For this review, take the finished solid that the model builds, in its own axes (mm). Face numbers are marked on the shaded views. A direction names the side the tool comes from. Round coordinates to 2 decimals unless told otherwise and drop trailing zeros. Loops run counter-clockwise (first coordinate to the right, second up) from the corner with the lowest first, then second, coordinate; pieces in that order, holes last. Notation, with made-up numbers: M 51.25,5.25 L 70.25,5.25 A22 cw 70.25,26.25 Z; hole C -25,43.25 d11. An arc over 180 degrees is marked long. Write item = value, one per line. Start each with the question number.
```python
from build123d import *

# Parameters (mm, degrees)
F0_R     = 3.78
F1_DEPTH = 6.88
F2_R     = 3.1
F3_DEPTH = 4.45
F4_R     = 2.5
F5_DEPTH = 11.6


# Not quite as in the source:
# - a fillet or chamfer that OpenCascade refuses, or shapes differently, is made with other operations: its cross-section is extruded or revolved along the edge and cut away or added


with BuildPart() as f1:
    # F0 (on Top) → F1 (new body)
    with BuildSketch(Plane.XY):
        Circle(F0_R)
    extrude(amount=F1_DEPTH)

    # F2 (on face) → F3 (join)
    with BuildSketch(Plane(origin=(0, 0, 0), x_dir=(1, 0, 0), z_dir=(0, 0, -1))):
        Circle(F2_R)
    extrude(amount=F3_DEPTH)

    # F4 (on face) → F5 (cut)
    with BuildSketch(Plane.XY.offset(6.88)):
        Circle(F4_R)
    extrude(amount=-F5_DEPTH, mode=Mode.SUBTRACT)

    # F6: chamfer of 1.4 on 1 edges, made by hand

    # F6_s1 → F6_t2 (revolve, cut)
    with BuildSketch(Plane.XZ):
        Polygon((3.78, 5.48), (2.38, 6.88), (3.78, 6.88), align=None)
    revolve(axis=Axis((0, 0, 6.88), (0, 0, 1)), mode=Mode.SUBTRACT)


solid = f1.part
```
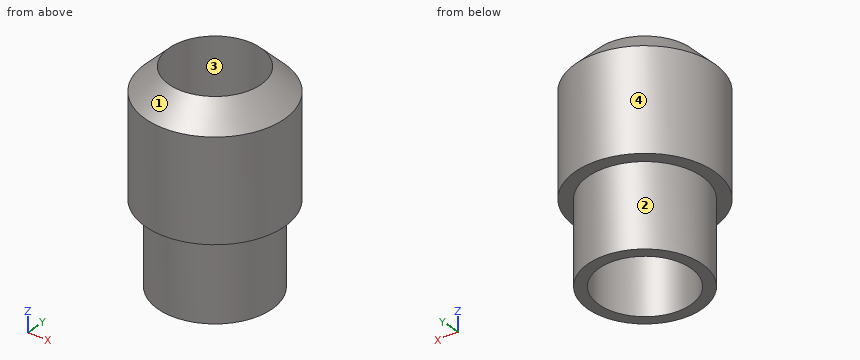
(1) Add section A-A on y = 0. Write out the cut boundary in (x, z).
(2) Wall thickness on L1, parallel to Y at x = 0, z = 3.25; L2, parallel to Y at x = 0, z = -1; L3, parallel to X at y = -2, z = 1.5: over which ranges is each line inside the solid? List them lowest first.
(3) For pin 1 Ø3 at (y, z) = (-2.5, 4.5) entering from +X; pin 2 Ø3 at (x, y) = (0, 0) entering from +Z; pin 3 Ø1.5 at (y, z) = (-3, -3.5) entering from -X, all flat-tipped, find the tip position at first contact; note any pin that passes through.
(4) Add section C-C on z = 3.5. Write out the cut boundary in (x, y), and give its area (3 significant figures).
(5) Add section D-D on z = -2.5. Write out the cut boundary in (x, y).
(6) Tool access review of the marked faces 1 and 2: name each direction out of +Z, -Z, +X, -X, +Y, -Y from which nothing blocks a thin tool from reaching the whole face with its end or side.
(7) Draft analysis for pull direction Y (two halves, no side actions). For the marked faces 3 and 4, state which applies: +Y half, -Y half, draft (parallel to the pull), parting line (faces both ways), or undercut.
Answer sheet:
q1.outline = M -3.78,0 L -3.1,0 L -3.1,-4.45 L -2.5,-4.45 L -2.5,6.76 L -3.78,5.48 Z; M 2.5,-4.45 L 3.1,-4.45 L 3.1,0 L 3.78,0 L 3.78,5.48 L 2.5,6.76 Z
q2.L1 = -3.78 to -2.5, 2.5 to 3.78
q2.L2 = -3.1 to -2.5, 2.5 to 3.1
q2.L3 = -3.21 to -1.5, 1.5 to 3.21
q3.pin_1 = 3.65
q3.pin_2 = through
q3.pin_3 = -2.13
q4.outline = C 0,0 d7.56; hole C 0,0 d5
q4.area = 25.3 mm²
q5.outline = C 0,0 d6.2; hole C 0,0 d5
q6.face_1 = +Z
q6.face_2 = -Z
q7.face_3 = undercut
q7.face_4 = parting line
